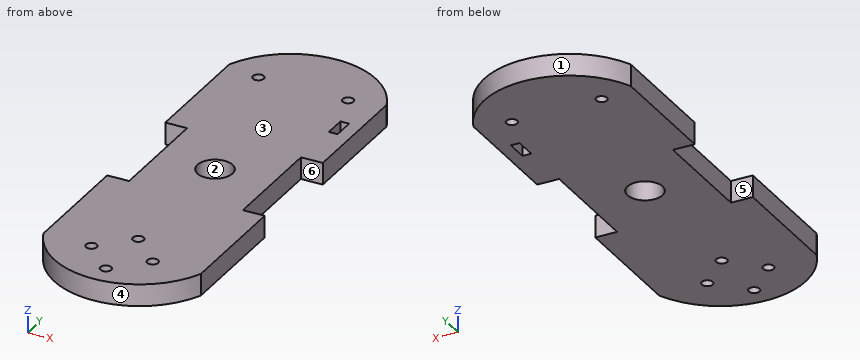
```python
from build123d import *

# Parameters (mm, degrees)
SKETCH1_R           = 1.25
SKETCH1_R_2         = 4
SKETCH1_W           = 2
SKETCH1_H           = 5
BOSS_EXTRUDE1_DEPTH = 5


with BuildPart() as part:
    # Sketch1 → Boss-Extrude1 (new body)
    with BuildSketch(Plane.XY):
        with BuildLine():
            Line((-18, 80), (-18, 52.5))
            Line((-18, 52.5), (-13, 52.5))
            Line((-13, 52.5), (-13, 27.5))
            Line((-13, 27.5), (-18, 27.5))
            Line((-18, 27.5), (-18, 0))
            ThreePointArc((-18, 0), (0, -12), (18, 0))
            Line((18, 0), (18, 27.5))
            Line((18, 27.5), (13, 27.5))
            Line((13, 27.5), (13, 52.5))
            Line((13, 52.5), (18, 52.5))
            Line((18, 52.5), (18, 80))
            ThreePointArc((18, 80), (0, 92), (-18, 80))
        make_face()
        with Locations((0, 7)):
            Circle(SKETCH1_R, mode=Mode.SUBTRACT)
        with Locations((7, 0)):
            Circle(SKETCH1_R, mode=Mode.SUBTRACT)
        with Locations((0, -7)):
            Circle(SKETCH1_R, mode=Mode.SUBTRACT)
        with Locations((-7, 0)):
            Circle(SKETCH1_R, mode=Mode.SUBTRACT)
        with Locations((0, 40)):
            Circle(SKETCH1_R_2, mode=Mode.SUBTRACT)
        with Locations((-10.25, 78)):
            Circle(SKETCH1_R, mode=Mode.SUBTRACT)
        with Locations((10.25, 78)):
            Circle(SKETCH1_R, mode=Mode.SUBTRACT)
        with Locations((14, 67)):
            Rectangle(SKETCH1_W, SKETCH1_H, mode=Mode.SUBTRACT)
    extrude(amount=BOSS_EXTRUDE1_DEPTH)


solid = part.part
```
Model file for the job. Use its own axes, mm. Face numbers are marked on the shaded views. A direction names the side the tool comes from. Coordinates: 2 decimals unless noted, no trailing zeros. Order: outer loops, then holes, each group sorted by start corner. A loop starts at its lowest first (then second) coordinate and runs counter-clockwise, first axis right, second up. Notation, with made-up numbers: (-34, 84) - (-6, 84) arc R23 ccw to (-6, 98) - close; hole circle Ø11 at (26.5, 83.5). An arc over 180 degrees is marked (long way). Return JSON: item names as keys, results as strings. Group by question number.
1) Saw through at A-A, the plane x = 0. Write the cut outline in (y, z), plus the area to 3 significant figures.
2) Probe line 1 (X direction, y = 78, z = 1.55); line 2 (Y direction, x = 0, z = 3.1); line 3 (X direction, y = 29, z = 4.6). List the from-to ranges inside material, lowest first. Write a range as from..to.
3) Mould opens along Y. For the marked faces 1, 2 and 3 say: released by +Y, released by -Y, zero draft, split by the parting line, or undercut.
4) Flat gauge pins, fed straight in: P1, Ø1.5, axis at y = 35, z = 2.5, coming from the +X side; P2, Ø3, axis at x = -7, y = 0, coming from the +Z side; P3, Ø2, axis at x = 14.5, z = 2, coming from the +Y side; P4, Ø1.6, axis at x = 13.5, z = 3, coming from the -Y side. Where does each tip first touch, or does it go through?
5) Saw through at C-C, the plane y = 7. Write the cut outline in (x, z), plus the area to 4 significant figures.
6) Saw through at D-D, the plane x = -7. Write the cut outline in (y, z).
7) Saw through at B-B, the plane z = 4.15. Count the separate pieces of the cut face and the enclosed holes in it, plus the area to 3 significant figures.
8) Tool access for the marked faces 4, 5 and 6: list every direction of +Z, -Z, +X, -X, +Y, -Y with a clear straight run to the whole face (end or side of a thin tool).
Values found:
{
 "1": {"outline": "(-12, 0) - (-8.25, 0) - (-8.25, 5) - (-12, 5) - close; (-5.75, 0) - (5.75, 0) - (5.75, 5) - (-5.75, 5) - close; (8.25, 0) - (36, 0) - (36, 5) - (8.25, 5) - close; (44, 0) - (92, 0) - (92, 5) - (44, 5) - close", "area": "455 mm²"},
 "2": {"line 1": "x = -18..-11.5, -9..9, 11.5..18", "line 2": "y = -12..-8.25, -5.75..5.75, 8.25..36, 44..92", "line 3": "x = -13..13"},
 "3": {"face 1": "released by +Y", "face 2": "undercut", "face 3": "zero draft"},
 "4": {"P1": "stops at x = 13", "P2": "stops at z = 5", "P3": "stops at y = 86.57", "P4": "stops at y = -7.3"},
 "5": {"outline": "(-18, 0) - (-1.25, 0) - (-1.25, 5) - (-18, 5) - close; (1.25, 0) - (18, 0) - (18, 5) - (1.25, 5) - close", "area": "167.5 mm²"},
 "6": {"outline": "(-10.7, 0) - (-1.25, 0) - (-1.25, 5) - (-10.7, 5) - close; (1.25, 0) - (90.7, 0) - (90.7, 5) - (1.25, 5) - close"},
 "7": {"separate pieces": "1", "enclosed holes": "8", "area": "3,160 mm²"},
 "8": {"face 4": "+Z, -Z, -Y", "face 5": "+Z, -Z, -X", "face 6": "+Z, -Z, +X"}
}
